The model under review builds one solid part; all positions refer to its coordinate system, in mm. Face numbers are marked on the shaded views. A direction names the side the tool comes from. Coordinates: 2 decimals unless noted, no trailing zeros. Order: outer loops, then holes, each group sorted by start corner. A loop starts at its lowest first (then second) coordinate and runs counter-clockwise, first axis right, second up. Notation, with made-up numbers: (19.5, 15) -> (58.5, 15) arc R30 cw to (58.5, 39) -> close; hole circle Ø5 at (-21.5, 37). An arc over 180 degrees is marked (long way). Use one line per item in the form item = value. Start each with the question number.
(1) Take a section at C-C (z = 37.5). State the section outline as (x, y) points (3 decimals).
(2) Mouldability with a two-part tool opening along Z and no side actions: class the marked faces 1, 2 and 3 as +Z half, -Z half, draft (parallel to the pull), parting line (faces both ways), or undercut.
(3) Wall thickness on line 1 along Z through (x, y) = (-14, 7); line 2 along X through (y, z) = (6.5, 31) (3 decimals); line 3 along X through (y, z) = (11, 0) (3 decimals): over which ranges is each line inside the solid? List them lowest first.
(4) Insertion check: pin 1 Ø4.5 at (x, z) = (28.575, 0) entering from +Y; pin 2 Ø7.5 at (x, z) = (33, -2) entering from -Y; pin 3 Ø5 at (x, z) = (14, -14.5) entering from +Y; pin 4 Ø8 at (y, z) = (12.5, -7.5) entering from +X. Each pin has a flat end and moves straight along its axis. Give the tip position at first contact, or say it passes through.
(5) Take a section at D-D (y = 20.5). State the section outline as (x, z) points (3 decimals).
(6) Take a section at A-A (z = 0). State the section outline as (x, y) points (3 decimals).
(7) For the marked faces 4, 5 and 6, list the 3-axis set-ups (+Z, -Z, +X, -X, +Y, -Y) from which the entire face can be reached by the end or side of a thin tool; tool diameter is ignored.
(8) Take a section at B-B (x = -7). State the section outline as (y, z) points, then the cut area to 3 significant figures.
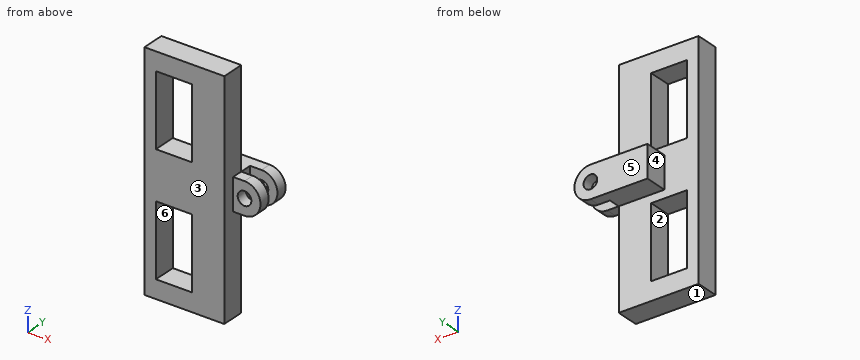
```python
from build123d import *

# Parameters (mm, degrees)
SKETCH1_W                = 44.45
SKETCH1_H                = 127
SKETCH1_W_2              = 20.060000012
SKETCH1_H_2              = 40.00000001
BOSS_EXTRUDE1_DEPTH      = 12.7
SKETCH2_R                = 3.81
BOSS_EXTRUDE2_DEPTH      = 12.7
BOSS_EXTRUDE2_DEPTH_BACK = 12.7
SKETCH3_W                = 15.24
SKETCH3_H                = 6.604
CUT_EXTRUDE1_DEPTH       = 23.114


with BuildPart() as part:
    # Sketch1 → Boss-Extrude1 (new body)
    with BuildSketch(Plane(origin=(0, 0, 0), x_dir=(1, 0, 0), z_dir=(0, 1, 0))):
        Rectangle(SKETCH1_W, SKETCH1_H)
        with Locations((-5.844999994, 33.339999995)):
            Rectangle(SKETCH1_W_2, SKETCH1_H_2, mode=Mode.SUBTRACT)
        with Locations((-5.844999994, -33.339999995)):
            Rectangle(SKETCH1_W_2, SKETCH1_H_2, mode=Mode.SUBTRACT)
    extrude(amount=BOSS_EXTRUDE1_DEPTH)

    # Sketch2 → Boss-Extrude2 (add, two sides)
    with BuildSketch(Plane(origin=(0, 12.7, 0), x_dir=(1, 0, 0), z_dir=(0, 1, 0))) as boss_extrude2_sk:
        with BuildLine():
            Line((28.575, 8.89), (-3.175, 8.89))
            Line((-3.175, 8.89), (-3.175, -8.89))
            Line((-3.175, -8.89), (28.575, -8.89))
            ThreePointArc((28.575, -8.89), (37.465, 0), (28.575, 8.89))
        make_face()
        with Locations((28.575, 0)):
            Circle(SKETCH2_R, mode=Mode.SUBTRACT)
    extrude(amount=BOSS_EXTRUDE2_DEPTH)
    extrude(boss_extrude2_sk.sketch, amount=-BOSS_EXTRUDE2_DEPTH_BACK)

    # Sketch3 → Cut-Extrude1 (cut)
    with BuildSketch(Plane.XY.offset(8.89)):
        with Locations((29.845, 16.002)):
            Rectangle(SKETCH3_W, SKETCH3_H)
        with Locations((29.845, 3.302)):
            Rectangle(SKETCH3_W, SKETCH3_H)
    extrude(amount=-CUT_EXTRUDE1_DEPTH, mode=Mode.SUBTRACT)


solid = part.part
```
Findings:
q1.outline = (-22.225, 0) -> (-15.875, 0) -> (-15.875, 12.7) -> (-22.225, 12.7) -> close; (4.185, 0) -> (22.225, 0) -> (22.225, 12.7) -> (4.185, 12.7) -> close
q2.face_1 = -Z half
q2.face_2 = undercut
q2.face_3 = draft
q3.line_1 = -63.5 to -53.34, -13.34 to 13.34, 53.34 to 63.5
q3.line_2 = -22.225 to -15.875, 4.185 to 22.225
q3.line_3 = -22.225 to 24.765, 32.385 to 37.465
q4.pin_1 = through
q4.pin_2 = 6.6
q4.pin_3 = 12.7
q4.pin_4 = 36.75
q5.outline = (-3.175, -8.89) -> (28.575, -8.89) arc R8.89 ccw to (28.575, 8.89) -> (-3.175, 8.89) -> close; hole circle Ø7.62 at (28.575, 0)
q6.outline = (-22.225, 0) -> (22.225, 0) -> (22.225, 6.604) -> (24.765, 6.604) -> (24.765, 12.7) -> (22.225, 12.7) -> (22.225, 19.304) -> (24.765, 19.304) -> (24.765, 25.4) -> (-3.175, 25.4) -> (-3.175, 12.7) -> (-22.225, 12.7) -> close; (32.385, 6.604) -> (37.465, 6.604) -> (37.465, 12.7) -> (32.385, 12.7) -> close; (32.385, 19.304) -> (37.465, 19.304) -> (37.465, 25.4) -> (32.385, 25.4) -> close
q7.face_4 = +Z, -Z, -X, +Y
q7.face_5 = +Z, -Z, +X, -X, +Y
q7.face_6 = +Y, -Y
q8.outline = (0, -63.5) -> (12.7, -63.5) -> (12.7, -53.34) -> (0, -53.34) -> close; (0, -13.34) -> (12.7, -13.34) -> (12.7, 13.34) -> (0, 13.34) -> close; (0, 53.34) -> (12.7, 53.34) -> (12.7, 63.5) -> (0, 63.5) -> close
q8.area = 597 mm²
